Work out the finished part from the listing and answer in its coordinate system (mm). A direction names the side the tool comes from. Coordinates: 2 decimals unless noted, no trailing zeros. Write each loop counter-clockwise with the first axis right and the second up, starting at its lowest first coordinate (ties: lowest second). Pieces come first, ordered by that corner, then holes. Notation, with made-up numbers: (34, -11.75) -> (59, -11.75) arc R27 cw to (59, 23.25) -> close; hole circle Ø3 at (58.5, 20). An arc over 180 degrees is marked (long way). Write each question's results on one line, items separated by ' | '. Start each with the question number.
from build123d import *

# Parameters (mm, degrees)
F0_R     = 38.1
F1_DEPTH = 12.7
F2_R     = 7.62
F3_DEPTH = 127
F6_DEPTH = 38.1


# Not quite as in the source:
# - a feature names something its author has since deleted; it is built from what else it names


with BuildPart() as f1:
    # F0 (on Top) → F1 (new body)
    with BuildSketch(Plane.XY):
        Circle(F0_R)
    extrude(amount=F1_DEPTH)

    # F2 (on face) → F3 (join)
    with BuildSketch(Plane.XY.offset(12.7)):
        Circle(F2_R)
    extrude(amount=F3_DEPTH)

    # F4 (on Right) → F5 (revolve)
    with BuildSketch(Plane.YZ):
        Polygon((0, 190.5), (0, 139.7), (7.62, 139.7), (3.81, 190.5), align=None)
    revolve(axis=Axis((0, 0, 165.1), (0, 0, 1)))

    # F6 (add): a face of the model
    f6_faces = [f1.faces().sort_by_distance(p)[0] for p in [
        (0, 0, 190.5),
    ]]
    extrude(f6_faces, amount=F6_DEPTH)


solid = f1.part
1. For faces 1 (the face through (0, 0, 228.6)), 2 (the face through (3.72, -0.83, 209.28)), determine the directions among +Z, -Z, +X, -X, +Y, -Y from which every point of the face is accessible in a straight line to the end or side of a thin tool.
2. Find section C-C on z = 48. Give the vertices of the cut face in (x, y), and give its area (3 significant figures).
3. Given pin 1 Ø1.5 at (x, y) = (8, 25) entering from +Z; pin 2 Ø10 at (y, z) = (3.5, 121) entering from +X; pin 3 Ø4 at (x, z) = (-3.5, 179) entering from +Y; pin 4 Ø1 at (y, z) = (-9.5, 119) entering from +X, each flat-ended and moving along its own axis, determine where each tip first touches the part or whether it passes through.
4. Find section A-A on y = 0. Give the vertices of the cut face in (x, z).
5. Find section D-D on x = 20.5. Give the vertices of the cut face in (y, z).
6. Find the intervals of material crossed by L1, parallel to Z at x = -22.5, y = 22.5; L2, parallel to Y at x = -0.5, z = 128; L3, parallel to X at y = 3, z = 154, in increasing order.
Ans:
1) face 1: +Z, +X, -X, +Y, -Y | face 2: +Z
2) outline: circle Ø15.24 at (0, 0) | area: 182 mm²
3) pin 1: stops at z = 12.7 | pin 2: stops at x = 7.62 | pin 3: stops at y = 4.44 | pin 4: passes through
4) outline: (-38.1, 0) -> (38.1, 0) -> (38.1, 12.7) -> (7.62, 12.7) -> (7.62, 139.7) -> (3.81, 190.5) -> (3.81, 228.6) -> (-3.81, 228.6) -> (-3.81, 190.5) -> (-7.62, 139.7) -> (-7.62, 12.7) -> (-38.1, 12.7) -> close
5) outline: (-32.11, 0) -> (32.11, 0) -> (32.11, 12.7) -> (-32.11, 12.7) -> close
6) L1: z = 0 to 12.7 | L2: y = -7.6 to 7.6 | L3: x = -5.82 to 5.82
